```python
from build123d import *

# Parameters (mm, degrees)
SKETCH1_R           = 2
SKETCH1_R_2         = 0.5
BOSS_EXTRUDE1_DEPTH = 2
BOSS_EXTRUDE2_START = 2
SKETCH1_3_R         = 2
BOSS_EXTRUDE2_DEPTH = 15


with BuildPart() as part:
    # Sketch1 → Boss-Extrude1 (new body)
    with BuildSketch(Plane(origin=(0, 0, 0), x_dir=(1, 0, 0), z_dir=(0, 1, 0))):
        with BuildLine():
            Line((2, 7.5), (2, 2.88735269))
            Line((2, 2.88735269), (17.117647059, 1.996536794))
            ThreePointArc((17.117647059, 1.996536794), (19, 0), (17.117647059, -1.996536794))
            Line((17.117647059, -1.996536794), (2, -2.88735269))
            Line((2, -2.88735269), (2, -7.5))
            ThreePointArc((2, -7.5), (0, -9.5), (-2, -7.5))
            Line((-2, -7.5), (-2, -2.88735269))
            Line((-2, -2.88735269), (-17.117647059, -1.996536794))
            ThreePointArc((-17.117647059, -1.996536794), (-19, 0), (-17.117647059, 1.996536794))
            Line((-17.117647059, 1.996536794), (-2, 2.88735269))
            Line((-2, 2.88735269), (-2, 7.5))
            ThreePointArc((-2, 7.5), (0, 9.5), (2, 7.5))
        make_face()
        Circle(SKETCH1_R, mode=Mode.SUBTRACT)
        with Locations((-17, 0)):
            Circle(SKETCH1_R_2, mode=Mode.SUBTRACT)
        with Locations((17, 0)):
            Circle(SKETCH1_R_2, mode=Mode.SUBTRACT)
        with Locations((-14.5, 0)):
            Circle(SKETCH1_R_2, mode=Mode.SUBTRACT)
        with Locations((-12, 0)):
            Circle(SKETCH1_R_2, mode=Mode.SUBTRACT)
        with Locations((-9.5, 0)):
            Circle(SKETCH1_R_2, mode=Mode.SUBTRACT)
        with Locations((-7, 0)):
            Circle(SKETCH1_R_2, mode=Mode.SUBTRACT)
        with Locations((-4.5, 0)):
            Circle(SKETCH1_R_2, mode=Mode.SUBTRACT)
        with Locations((4.5, 0)):
            Circle(SKETCH1_R_2, mode=Mode.SUBTRACT)
        with Locations((7, 0)):
            Circle(SKETCH1_R_2, mode=Mode.SUBTRACT)
        with Locations((9.5, 0)):
            Circle(SKETCH1_R_2, mode=Mode.SUBTRACT)
        with Locations((12, 0)):
            Circle(SKETCH1_R_2, mode=Mode.SUBTRACT)
        with Locations((14.5, 0)):
            Circle(SKETCH1_R_2, mode=Mode.SUBTRACT)
        with Locations((0, 7.5)):
            Circle(SKETCH1_R_2, mode=Mode.SUBTRACT)
        with Locations((0, 4.5)):
            Circle(SKETCH1_R_2, mode=Mode.SUBTRACT)
        with Locations((0, -4.5)):
            Circle(SKETCH1_R_2, mode=Mode.SUBTRACT)
        with Locations((0, -7.5)):
            Circle(SKETCH1_R_2, mode=Mode.SUBTRACT)
    extrude(amount=BOSS_EXTRUDE1_DEPTH)

    # Sketch1<3> → Boss-Extrude2 (add)
    with BuildSketch(Plane(origin=(0, 0, 0), x_dir=(1, 0, 0), z_dir=(0, 1, 0)).offset(BOSS_EXTRUDE2_START)):
        Circle(SKETCH1_3_R)
    extrude(amount=-BOSS_EXTRUDE2_DEPTH)


solid = part.part
```
Here's how the part is built. I have some questions about the finished solid (model axes, mm). A direction names the side the tool comes from. Give positions to 0.01 mm unless a question says otherwise; leave off trailing zeros. Order: outer loops, then holes, each group sorted by start corner. A loop starts at its lowest first (then second) coordinate and runs counter-clockwise, first axis right, second up. Notation, with made-up numbers: M 65.25,-24.75 L 96.25,-24.75 A17 ccw 96.25,-17.75 Z; hole C 38,-26 d4. An arc over 180 degrees is marked long. Use a Markdown table: item, result. Add a question column.
1. Suppose I cut it at B-B (x = -14.5). List the corners of the cut face in (y, z) for me.
2. Suppose I cut it at D-D (y = -5). List the corners of the cut face in (x, z) for me, and give its area (3 significant figures).
3. Suppose I cut it at C-C (z = 5.75). List the corners of the cut face in (x, y) for me, and give its area (3 significant figures).
4. For pin 1 Ø5 at (x, y) = (3.5, -8.5) entering from -Z; pin 2 Ø2 at (y, z) = (0.5, -6.5) entering from -X; pin 3 Ø1 at (y, z) = (1, 5) entering from +X; pin 4 Ø3 at (x, y) = (5, -2) entering from +Z (1 decimal), each with a flat end and sliding along its axis, tell me the tip position at first contact or that it passes through.
5. Suppose I cut it at A-A (z = -4.5). List the corners of the cut face in (x, y) for me, and give its area (3 significant figures).
6. On a 3-axis mill with a long thin cutter (end or side, diameter ignored), from which of +Z, -Z, +X, -X, +Y, -Y can I reach the whole of each face in a straight line? I mean faces 5 (the cylindrical face through (15, 1, 0)), 6 (the flat face through (2, 1, 5)). Say none if no direction works.
7. I need wall thicknesses on probe 1 along X at (y, z) = (0.4, -7.5); probe 2 along Y at (x, z) = (-6, 1); probe 3 along Z at (x, y) = (9.5, 1.65). Which ranges of each line are inside material? Lowest first, please. Write a range as from..to.
8. If we mould it in two halves opening along X, with no side actions, what happens to faces 1 (the flat face through (-9.665, 0.986, -2.436)), 2 (the cylindrical face through (-5, 1, 0)), 3 (the flat face through (9.45, 0.99, -2.45)), 4 (the cylindrical face through (4, 1, 0))? For each: +X half, -X half, draft (parallel to the pull), parting line (faces both ways), or undercut.
Results list:
| question | item | result |
|---|---|---|
| 1 | outline | M 0,-2.15 L 2,-2.15 L 2,-0.5 L 0,-0.5 Z; M 0,0.5 L 2,0.5 L 2,2.15 L 0,2.15 Z |
| 2 | outline | C 0,0 d4 |
| 2 | area | 12.6 mm² |
| 3 | outline | M -2,0 L 2,0 L 2,2 L -2,2 Z |
| 3 | area | 8.00 mm² |
| 4 | pin 1 | stops at z = -1.73 |
| 4 | pin 2 | stops at x = -2 |
| 4 | pin 3 | stops at x = 2 |
| 4 | pin 4 | passes through |
| 5 | outline | M -2,0 L -0.5,0 L -0.5,2 L -2,2 Z; M 0.5,0 L 2,0 L 2,2 L 0.5,2 Z |
| 5 | area | 6.00 mm² |
| 6 | face 5 | +Y, -Y |
| 6 | face 6 | +Z, +X, +Y, -Y |
| 7 | probe 1 | x = -2..-0.5, 0.5..2 |
| 7 | probe 2 | y = 0..2 |
| 7 | probe 3 | z = -2.45..-0.5, 0.5..2.45 |
| 8 | face 1 | -X half |
| 8 | face 2 | undercut |
| 8 | face 3 | +X half |
| 8 | face 4 | undercut |
